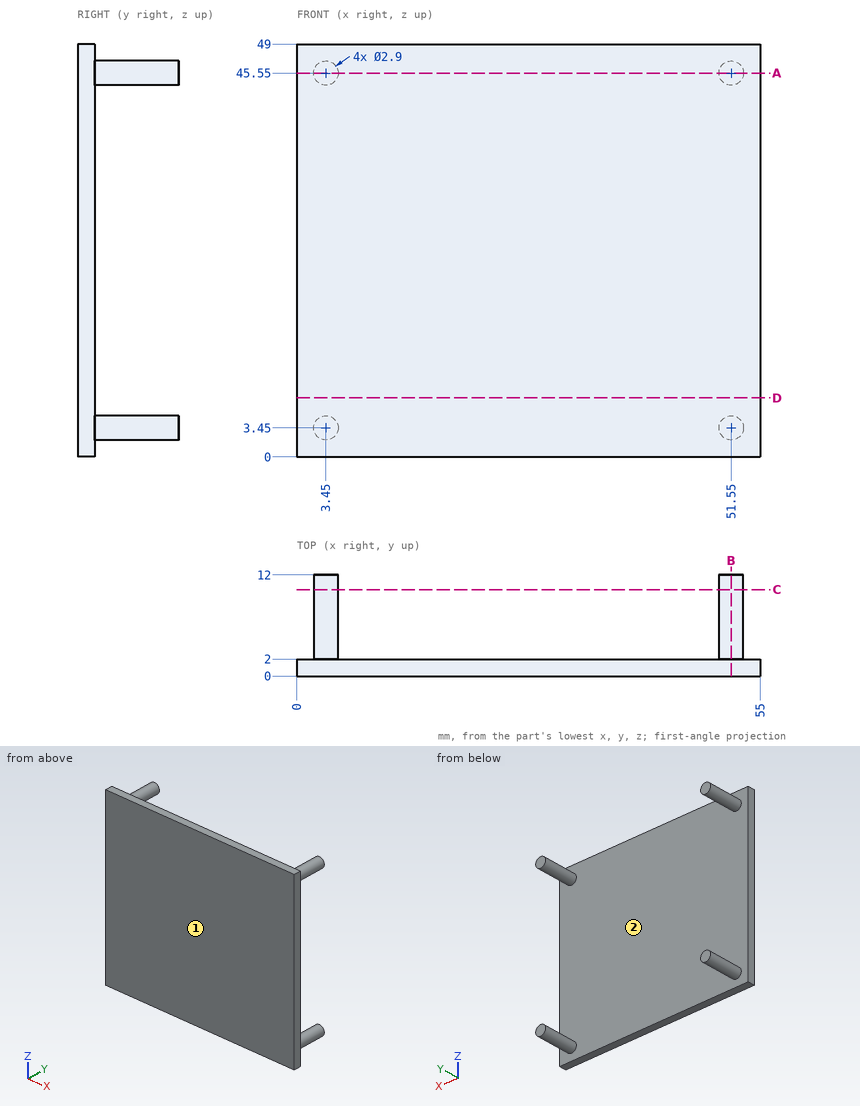
Study the drawing (mm; zero at the part's minimum x, y, z) and answer. A direction names the side the tool comes from. Give positions to 0.01 mm unless a question says otherwise; leave off trailing zeros. Order: outer loops, then holes, each group sorted by start corner. A loop starts at its lowest first (then second) coordinate and runs counter-clockwise, first axis right, second up. Notation, with made-up numbers: (54, 88) - (69, 88) arc R34 ccw to (69, 118) - close; hole circle Ø2 at (64.5, 65.25). An arc over 180 degrees is marked (long way). Use one line per item in the form item = value. Start each with the question number.
(1) Flat-ended cylindrical pins translate along their axes: pin 1 Ø6 at (y, z) = (4, 17) entering from -X; pin 2 Ø2 at (x, z) = (29.5, 8) entering from +Y. Find the tip coordinate at first contact, or state that the pin passes through.
(2) A cutting plane is placed at C-C, the plane y = 10.25. Write down the section's boundary in (x, z).
(3) A cutting plane is placed at D-D, the plane z = 7. Write down the section's boundary in (x, y).
(4) A cutting plane is placed at A-A, the plane z = 45.55. Write down the section's boundary in (x, y).
(5) Consider line 1 (Y direction, x = 10.5, z = 46); line 2 (Z direction, x = 3, y = 2.5). Determine where each line is inside the solid, lowest interval first. Write a range as from..to.
(6) A cutting plane is placed at B-B, the plane x = 51.55. Write down the section's boundary in (y, z).
(7) For the marked faces 1 and 2, determine the directions among +Z, -Z, +X, -X, +Y, -Y from which every point of the face is accessible in a straight line to the end or side of a thin tool.
Ans:
q1.pin_1 = 0
q1.pin_2 = 2
q2.outline = circle Ø2.9 at (3.45, 3.45); circle Ø2.9 at (3.45, 45.55); circle Ø2.9 at (51.55, 3.45); circle Ø2.9 at (51.55, 45.55)
q3.outline = (0, 0) - (55, 0) - (55, 2) - (0, 2) - close
q4.outline = (0, 0) - (55, 0) - (55, 2) - (53, 2) - (53, 12) - (50.1, 12) - (50.1, 2) - (4.9, 2) - (4.9, 12) - (2, 12) - (2, 2) - (0, 2) - close
q5.line_1 = 0..2
q5.line_2 = 2.07..4.83, 44.17..46.93
q6.outline = (0, 0) - (2, 0) - (2, 2) - (12, 2) - (12, 4.9) - (2, 4.9) - (2, 44.1) - (12, 44.1) - (12, 47) - (2, 47) - (2, 49) - (0, 49) - close
q7.face_1 = +Z, -Z, +X, -X, -Y
q7.face_2 = +Y
